The model under review builds one solid part; all positions refer to its coordinate system, in mm. Face numbers are marked on the shaded views. A direction names the side the tool comes from. Give positions to 0.01 mm unless a question says otherwise; leave off trailing zeros. Write each loop counter-clockwise with the first axis right and the second up, starting at its lowest first coordinate (ties: lowest second). Pieces come first, ordered by that corner, then holes.
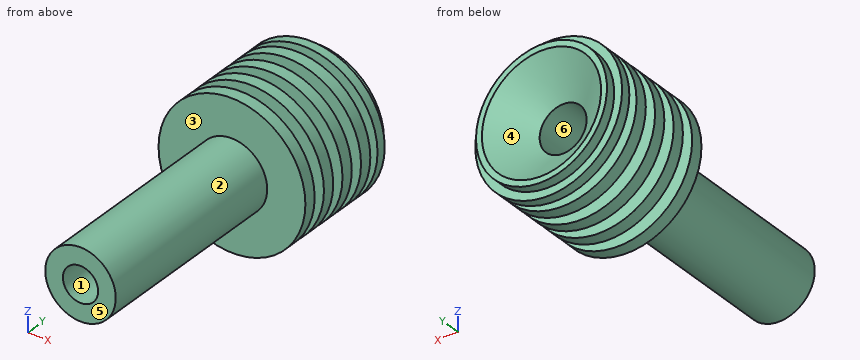
Autodesk Inventor part; units mm, degrees
ref_plane "Plano de trabajo3" through (0, 7.5, 0) normal (0, 1, 0) x (1, 0, 0)
ref_plane "Plano de trabajo17" through (0, 43.5716, 0) normal (0, -1, 0) x (1, 0, 0)
ref_plane "Plano de trabajo18" through (0, 49.9998, 0) normal (0, 1, 0) x (1, 0, 0)
sketch "Boceto1" plane through (0, 0, 0) normal (0, 1, 0) x (-1, 0, 0)
  circle A0 centre (0, 0) radius 6
  circle A1 centre (0, 0) radius 3
  dimension "d0" = 12
  dimension "d1" = 6
extrude "Extrusión1" add sketch "Boceto1" along normal blind 50
ref_plane "Plano de trabajo3" through (0, 7.5, 0) normal (0, 1, 0) x (1, 0, 0)
sketch "Boceto20" plane through (0, 50, 0) normal (0, 1, 0) x (1, 0, 0)
  circle A0 centre (0, 0) radius 7.75
  circle A1 centre (0, 0) radius 3.9641
  circle A2 centre (0, 0) radius 4
  dimension "d50" = 15.5
  dimension "d72" = 8
extrude "Extrusión14" add sketch "Boceto20" along normal blind 1.6666 contours A0
sketch "Boceto21" plane through (0, 51.6666, 0) normal (0, 1, 0) x (1, 0, 0)
  circle A0 centre (0, 0) radius 12.5
  circle A1 centre (0, 0) radius 4
  dimension "d53" = 25
extrude "Extrusión15" add sketch "Boceto21" along normal blind 1.6666
sketch "Boceto22" plane through (0, 53.3332, 0) normal (0, 1, 0) x (1, 0, 0)
  circle A0 centre (0, 0) radius 11.15
  circle A1 centre (0, 0) radius 3.9641
  dimension "d56" = 22.3
extrude "Extrusión16" add sketch "Boceto22" along normal blind 1.6666
ref_plane "Plano de trabajo17" through (0, 43.5716, 0) normal (0, -1, 0) x (1, 0, 0)
ref_plane "Plano de trabajo16" through (0, 41.4287, 0) normal (0, -1, 0) x (1, 0, 0)
sketch "Boceto23" plane through (0, 35, 0) normal (0, -1, 0) x (1, 0, 0)
  circle A0 centre (0, 0) radius 12.5
  circle A1 centre (0, 0) radius 6
  dimension "d64" = 25
  dimension "d65" = 12
extrude "Extrusión17" add sketch "Boceto23" against normal blind 2.1429
pattern_linear "Patrón rectangular1" count 4 spacing 4.2858 along (0, 1, 0) of "Extrusión17"
sketch "Boceto24" plane through (0, 54.9998, 0) normal (0, 1, 0) x (1, 0, 0)
  circle A0 centre (0, 0) radius 10.15
  dimension "d71" = 20.3
ref_plane "Plano de trabajo18" through (0, 49.9998, 0) normal (0, 1, 0) x (1, 0, 0)
sketch "Boceto25" plane through (0, 49.9998, 0) normal (0, 1, 0) x (1, 0, 0)
  circle A0 centre (0, 0) radius 4
  dimension "d74" = 8
loft "Solevación2" cut profiles "Boceto24", "Boceto25"
ref_plane "Plano de trabajo19" through (0, 7.5, 0) normal (0, -1, 0) x (1, 0, 0)
sketch "Boceto26" plane through (0, 7.5, 0) normal (0, -1, 0) x (1, 0, 0)
  circle A0 centre (0, 0) radius 6
  circle A1 centre (0, 0) radius 4
  dimension "d80" = 8
extrude "Extrusión18" cut sketch "Boceto26" against normal blind 47.5 contours A1
ref_plane "Plano de trabajo13" through (0, 35, 0) normal (0, -1, 0) x (1, 0, 0)
ref_plane "Plano de trabajo14" through (0, 37.1429, 0) normal (0, -1, 0) x (1, 0, 0)
ref_plane "Plano de trabajo15" through (0, 39.2858, 0) normal (0, -1, 0) x (1, 0, 0)
properties part number "Barrel husillo 8mm_V2"
1) Consider section A-A, the plane y = 10. Give the boundary of the cut face in (x, z), then the cut area to 3 significant figures.
2) To check wall thickness, follow probe 1 along Y at (x, z) = (10.25, -0.75); probe 2 along Y at (x, z) = (8.75, 7.75); probe 3 along Y at (x, z) = (6, -4.25). State the ranges of each line that lie inside material, in increasing order.
3) Insertion check: pin 1 (6.5 mm diameter, centred on x = -1, z = -0.5, fed in from +Y); pin 2 (5 mm diameter, centred on x = -3, y = 35, fed in from +Z); pin 3 (1.5 mm diameter, centred on x = -1, y = 28, fed in from -Z); pin 4 (3.5 mm diameter, centred on x = 0, z = 0, fed in from +Y). Each pin has a flat end and moves straight along its axis. Give the tip position at first contact, or say it passes through.
4) The part is to be moulded in two halves that separate along Z. For the marked faces 1, 2, 3 and 4, say which applies: +Z half, -Z half, draft (parallel to the pull), parting line (faces both ways), or undercut.
5) Consider section B-B, the plane z = -7. State how many separate pieces and enclosed holes the cut face has, then the cut area to 3 significant figures.
6) Tool access review of the marked faces 5 and 6: name each direction out of +Z, -Z, +X, -X, +Y, -Y from which nothing blocks a thin tool from reaching the whole face with its end or side.
Answer block:
1. outline: circle Ø12 at (0, 0); hole circle Ø8 at (0, 0)
1. area: 62.8 mm2
2. probe 1: y = 35 to 37.14, 39.29 to 41.43, 43.57 to 45.71, 47.86 to 50, 51.67 to 55
2. probe 2: y = 35 to 37.14, 39.29 to 41.43, 43.57 to 45.71, 47.86 to 50, 51.67 to 53.33
2. probe 3: y = 35 to 37.14, 39.29 to 41.43, 43.57 to 45.71, 47.86 to 52.73
3. pin 1: stops at y = 50.3
3. pin 2: stops at z = 12.49
3. pin 3: stops at z = -5.99
3. pin 4: passes through
4. face 1: undercut
4. face 2: parting line
4. face 3: draft
4. face 4: undercut
5. separate pieces: 4
5. enclosed holes: 0
5. area: 228 mm2
6. face 5: +Z, -Z, +X, -X, -Y
6. face 6: +Y
